Could you check a few things on this model? Use its own coordinates, in mm. A direction names the side the tool comes from. Coordinates: 2 decimals unless noted, no trailing zeros. Loops run counter-clockwise (first coordinate to the right, second up) from the corner with the lowest first, then second, coordinate; pieces in that order, holes last. Notation, with made-up numbers: (25, 37) - (57, 37) arc R26 ccw to (57, 75) - close; hole circle Ø5 at (56, 76). An arc over 180 degrees is marked (long way). One line per question, with ' | ' between items. Start each with the question number.
1. Which directions (+Z, -Z, +X, -X, +Y, -Y) give clear straight access to the entire face, cutting with the end or side of a thin tool? Please do faces 1 (the cylindrical face through (-7.72, -2.54, 2.1)), 2 (the conical face through (-6.072, -4.014, 1.651)), 3 (the flat face through (-3.122, -1.979, -5.407)).
2. I want a section at A-A, the plane y = 16. Write out the boundary of the cut face in (x, z), then the cut area to 3 significant figures.
3. Please list where these lines run through material, in increasing order: L1, parallel to Y at x = 3.25, z = -4.75; L2, parallel to Z at x = -0.25, y = 16; L3, parallel to X at y = 6, z = -6. Write a range as [from, to].
4. We'd pull the mould along Z, two halves only. Please class faces 4 (the cylindrical face through (-5.678, -2.535, -5.636)), 5 (the cylindrical face through (-2.042, -2.535, 7.735)), 6 (the cylindrical face through (-0.54, -2.46, 2.44)): pulls with the +Z half, pulls with the -Z half, needs draft (parallel to the pull), parting line crosses it, or undercut.
5. I'm going to push flat-ended pins straight in: P1, Ø3, axis at x = 7.5, y = 25, coming from the -Z side; P2, Ø1, axis at y = -3, z = -5.5, coming from the -X side (3 decimals); P3, Ø1.5, axis at x = -1, y = 14.5, coming from the -Z side. Where does each tip first touch, or does it pass through?
Autodesk Inventor part; units mm, degrees
ref_plane "Work Plane1" through (0, -5, 8) normal (1, 0, 0) x (0, 0, -1)
ref_plane "Work Plane2" through (10, 0, 0) normal (1, 0, 0) x (0, 1, 0)
ref_plane "XZ Plane" through (0, 0, 0) normal (0, 1, 0) x (-1, 0, 0)
sketch "Sketch1" plane through (0, 0, 0) normal (0, 1, 0) x (-1, 0, 0)
  circle A0 centre (0, 0) radius 10
  dimension "d0" = 20
extrude "Extrusion1" add sketch "Sketch1" along normal blind 30
sketch "Sketch2" plane through (0, 0, 0) normal (0, -1, 0) x (1, 0, 0)
  circle A0 centre (0, 0) radius 2.5
  dimension "d3" = 5
extrude "Extrusion2" add sketch "Sketch2" along normal blind 5
sketch "Sketch3" plane through (0, -5, 0) normal (0, -1, 0) x (1, 0, 0)
  circle A0 centre (0, 0) radius 2.5
  circle A1 centre (0, 0) radius 4.536
  circle A2 centre (0, 0) radius 8
  line L0 (0, -4.536) -> (0, -8)
  line L1 (0, 0) -> (4, -6.9282)
  line L2 (0, 0) -> (8, 0) construction
  point P0 (2.268, -3.9283)
  dimension "d6" = 9.072
  dimension "d7" = 16
  dimension "d8" = 60
extrude "Extrusion3" add sketch "Sketch3" against normal blind 5 contours L1 A2 L0 A1 picked at (1.6377, -6.621)
pattern_circular "Circular Pattern1" count 6 over 360 about axis through (0, 0, 0) along (0, -1, 0) of "Extrusion3"
ref_plane "Work Plane1" through (0, -5, 8) normal (1, 0, 0) x (0, 0, -1)
sketch "Sketch4" plane through (0, -5, 8) normal (1, 0, 0) x (0, 0, -1)
  line L0 (0, 0) -> (1.0718, 0)
  line L1 (0, 0) -> (3.4641, 2)
  line L2 (0, 0) -> (4, 0) construction
  line L3 (0, 0) -> (3.4641, 0)
  line L4 (3.4641, 2) -> (3.4641, 0)
  line L5 (5.732, 0) -> (5.732, 5)
  line L6 (8, -7) -> (8, 42)
  point P0 (8, 5)
  dimension "d15" = 4
  dimension "d16" = 30
revolve "Revolution1" cut sketch "Sketch4" angle 360 about axis through (0, -10, 0) along (0, -1, 0)
ref_plane "Work Plane2" through (10, 0, 0) normal (1, 0, 0) x (0, 1, 0)
properties part number "pot gövde"
Results are:
1) face 1: +Z, -X, -Y | face 2: -Y | face 3: -Z, -Y
2) outline: circle Ø20 at (0, 0) | area: 314 mm2
3) L1: y = [0, 30] | L2: z = [-10, 10] | L3: x = [-8, 8]
4) face 4: pulls with the -Z half | face 5: pulls with the +Z half | face 6: undercut
5) P1: stops at z = -8 | P2: stops at x = -6.245 | P3: stops at z = -10
